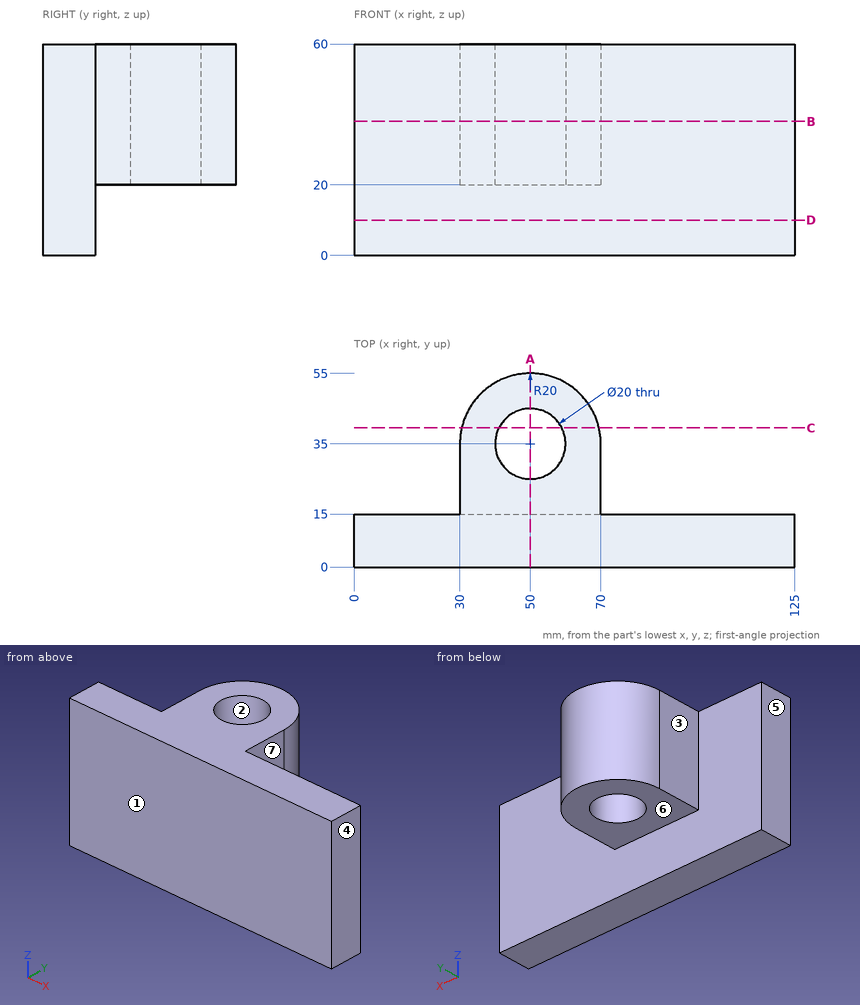
Answer from the drawing. Dimensions are ordinates in mm from the lowest x, y and z of the part. A direction names the side the tool comes from. Coordinates: 2 decimals unless noted, no trailing zeros. Loops run counter-clockwise (first coordinate to the right, second up) from the corner with the lowest first, then second, coordinate; pieces in that order, holes last. Notation, with made-up numbers: (-10.75, -38) - (14.25, -38) arc R17 cw to (14.25, -7) - close; hole circle Ø1 at (50.25, 47.25). An arc over 180 degrees is marked (long way). Answer in a Markdown table with one row per item.
1. Find section A-A, the plane x = 50. Write down the section's boundary in (y, z).
Conclusion:
| item | result |
|---|---|
| outline | (0, 0) - (15, 0) - (15, 20) - (25, 20) - (25, 60) - (0, 60) - close; (45, 20) - (55, 20) - (55, 60) - (45, 60) - close |
2. Find section C-C, the plane y = 39.5. Write down the section's boundary in (x, z), then the cut area to 3 significant figures.
Conclusion:
| item | result |
|---|---|
| outline | (30.51, 20) - (41.07, 20) - (41.07, 60) - (30.51, 60) - close; (58.93, 20) - (69.49, 20) - (69.49, 60) - (58.93, 60) - close |
| area | 845 mm² |
3. Which of the six approach directions +Z, -Z, +X, -X, +Y, -Y give full straight-line access (tool end or side, diameter ignored) to the marked faces 5, 6 and 7?
Conclusion:
| item | result |
|---|---|
| face 5 | +Z, -Z, -X, +Y, -Y |
| face 6 | -Z, +X, -X, +Y |
| face 7 | +Z, -Z, +X, +Y |
4. Determine the mould class of the marked faces 1, 2, 3 and 4 for opening direction X: +X half, -X half, draft (parallel to the pull), parting line (faces both ways), or undercut.
Conclusion:
| item | result |
|---|---|
| face 1 | draft |
| face 2 | undercut |
| face 3 | -X half |
| face 4 | +X half |
5. Given pin 1 (10 mm diameter, centred on y = 26.5, z = 35.5, fed in from +X); pin 2 (1 mm diameter, centred on y = 16.5, z = 42.5, fed in from -X); pin 3 (16 mm diameter, centred on y = 22, z = 40, fed in from -X); pin 4 (1 mm diameter, centred on x = 76.5, z = 19, fed in from +Y), each flat-ended and moving along its own axis, determine where each tip first touches the part or whether it passes through.
Conclusion:
| item | result |
|---|---|
| pin 1 | stops at x = 70 |
| pin 2 | stops at x = 30 |
| pin 3 | stops at x = 0 |
| pin 4 | stops at y = 15 |
6. Find section D-D, the plane z = 10. Write down the section's boundary in (x, y).
Conclusion:
| item | result |
|---|---|
| outline | (0, 0) - (125, 0) - (125, 15) - (0, 15) - close |
7. Find section B-B, the plane z = 38. Write down the section's boundary in (x, y), then the cut area to 3 significant figures.
Conclusion:
| item | result |
|---|---|
| outline | (0, 0) - (125, 0) - (125, 15) - (70, 15) - (70, 35) arc R20 ccw to (30, 35) - (30, 15) - (0, 15) - close; hole circle Ø20 at (50, 35) |
| area | 2,990 mm² |
8. Straight lines are drawn through the part: line 1 (Y direction, x = 50, z = 42); line 2 (Y direction, x = 86.5, z = 23.5); line 3 (X direction, y = 16, z = 32). For each, find the intervals that lie inside material, in ascending order.
Conclusion:
| item | result |
|---|---|
| line 1 | y = 0 to 25, 45 to 55 |
| line 2 | y = 0 to 15 |
| line 3 | x = 30 to 70 |
